Work out the finished part from the listing and answer in its coordinate system (mm). A direction names the side the tool comes from. Round coordinates to 2 decimals unless told otherwise and drop trailing zeros. Write each loop counter-clockwise with the first axis right and the second up, starting at its lowest first coordinate (ties: lowest second). Pieces come first, ordered by that corner, then holes. Notation, with made-up numbers: M 58,9.5 L 84,9.5 A20 ccw 84,22.5 Z; hole C -38.5,31 d4. An arc over 180 degrees is marked long. Answer in a Markdown table with one row per item.
```python
from build123d import *

# Parameters (mm, degrees)
SKETCH_1_W      = 2.5
SKETCH_1_H      = 2.5
EXTRUDE_1_DEPTH = 3
SKETCH_3_R      = 0.9
EXTRUDE_2_DEPTH = 1
SKETCH_4_R      = 0.3
EXTRUDE_3_DEPTH = 3
SKETCH_5_R      = 0.25
EXTRUDE_4_DEPTH = 5
CHAMFER_1_SIZE  = 0.5
CHAMFER_1_SIZE2 = 0.866025404


with BuildPart() as part:
    # Эскиз1 → Бобышка-Вытянуть1 (new body)
    with BuildSketch(Plane(origin=(0, 0, 0), x_dir=(1, 0, 0), z_dir=(0, 1, 0))):
        Rectangle(SKETCH_1_W, SKETCH_1_H)
    extrude(amount=EXTRUDE_1_DEPTH)

    # Эскиз3 → Бобышка-Вытянуть2 (add)
    with BuildSketch(Plane.XZ):
        with Locations(Location((0, 0, 0), (0, 0, 270))):
            Circle(SKETCH_3_R)
    extrude(amount=EXTRUDE_2_DEPTH)

    # Эскиз4 → Бобышка-Вытянуть3 (add)
    with BuildSketch(Plane.XZ.offset(1)):
        with Locations(Location((0, 0, 0), (0, 0, 270))):
            Circle(SKETCH_4_R)
    extrude(amount=EXTRUDE_3_DEPTH)

    # Эскиз5 → Бобышка-Вытянуть4 (add)
    with BuildSketch(Plane(origin=(0, 3, 0), x_dir=(1, 0, 0), z_dir=(0, 1, 0))):
        with Locations(Location((0, 0, 0), (0, 0, 90))):
            Circle(SKETCH_5_R)
    extrude(amount=EXTRUDE_4_DEPTH)

    # Фаска1
    chamfer_1_edges = [part.edges().sort_by_distance(p)[0] for p in [
        (0, 3, 0.25),
    ]]
    chamfer_1_side = [part.faces().sort_by_distance(p)[0] for p in [
        (0, 3, -1.214644661),
    ]]
    chamfer(chamfer_1_edges, length=CHAMFER_1_SIZE, length2=CHAMFER_1_SIZE2, reference=chamfer_1_side[0])


solid = part.part
```
1. Consider line 1 along Y through (x, z) = (-0.7, -0.35); line 2 along Y through (x, z) = (0.7, 0.85); line 3 along Z through (x, y) = (-0.1, 3.5). Determine where each line is inside the solid, lowest interval first. Write a range as from..to.
Calculated:
| item | result |
|---|---|
| line 1 | y = -1..3 |
| line 2 | y = 0..3 |
| line 3 | z = -0.45..0.45 |
2. A tool of negligible diameter and unlimited length cuts with its end or side. For faces 1 (the cylindrical face through (-0.345, -0.493, -0.831)), 2 (the flat face through (0, 1, 1.25)), 3 (the flat face through (1, 3, -1)), from which of +Z, -Z, +X, -X, +Y, -Y can it reach the whole face along a straight path? Write none if from no direction.
Calculated:
| item | result |
|---|---|
| face 1 | -Y |
| face 2 | +Z, +X, -X, +Y, -Y |
| face 3 | +Y |
3. The part is cut by section C-C (y = -2). Determine the outline of the cut face in (x, z), plus the area to 3 significant figures.
Calculated:
| item | result |
|---|---|
| outline | C 0,0 d0.6 |
| area | 0.283 mm² |
4. The part is cut by section B-B (z = 0). Determine the outline of the cut face in (x, y).
Calculated:
| item | result |
|---|---|
| outline | M -1.25,0 L -0.9,0 L -0.9,-1 L -0.3,-1 L -0.3,-4 L 0.3,-4 L 0.3,-1 L 0.9,-1 L 0.9,0 L 1.25,0 L 1.25,3 L 0.75,3 L 0.25,3.87 L 0.25,8 L -0.25,8 L -0.25,3.87 L -0.75,3 L -1.25,3 Z |
5. The part is cut by section D-D (y = 5). Determine the outline of the cut face in (x, z), plus the area to 3 significant figures.
Calculated:
| item | result |
|---|---|
| outline | C 0,0 d0.5 |
| area | 0.196 mm² |
6. The part is cut by section A-A (x = 0). Determine the outline of the cut face in (y, z), plus the area to 3 significant figures.
Calculated:
| item | result |
|---|---|
| outline | M -4,-0.3 L -1,-0.3 L -1,-0.9 L 0,-0.9 L 0,-1.25 L 3,-1.25 L 3,-0.75 L 3.87,-0.25 L 8,-0.25 L 8,0.25 L 3.87,0.25 L 3,0.75 L 3,1.25 L 0,1.25 L 0,0.9 L -1,0.9 L -1,0.3 L -4,0.3 Z |
| area | 14.0 mm² |
